```python
from build123d import *

# Parameters (mm, degrees)
FR4_DEPTH                     = 1.7526
SKETCH6_W                     = 5.5
SKETCH6_H                     = 5
SKETCH6_W_2                   = 13.6
SKETCH6_H_2                   = 5.5
FIBER_TRANSCEIVER_SLOTS_DEPTH = 143.1375095
SKETCH7_R                     = 1.905
CUT_EXTRUDE1_DEPTH            = 143.1375095
SKETCH8_R                     = 3.175
CUT_EXTRUDE2_DEPTH            = 143.1375095
CUT_EXTRUDE3_DEPTH            = 143.1375095


with BuildPart() as part:
    # Sketch1 → FR4 (new body)
    with BuildSketch(Plane(origin=(0, 0, 0), x_dir=(1, 0, 0), z_dir=(0, 1, 0))):
        with BuildLine():
            Line((0, 0), (5, 0))
            ThreePointArc((5, 0), (6.414213562, -0.585786438), (7, -2))
            Line((7, -2), (7, -13))
            ThreePointArc((7, -13), (7.585786438, -14.414213562), (9, -15))
            Line((9, -15), (22.5, -15))
            ThreePointArc((22.5, -15), (23.914213562, -14.414213562), (24.5, -13))
            Line((24.5, -13), (24.5, -2))
            ThreePointArc((24.5, -2), (25.085786438, -0.585786438), (26.5, 0))
            Line((26.5, 0), (83.5, 0))
            ThreePointArc((83.5, 0), (84.914213562, -0.585786438), (85.5, -2))
            Line((85.5, -2), (85.5, -13))
            ThreePointArc((85.5, -13), (86.085786438, -14.414213562), (87.5, -15))
            Line((87.5, -15), (101, -15))
            ThreePointArc((101, -15), (102.414213562, -14.414213562), (103, -13))
            Line((103, -13), (103, -2))
            ThreePointArc((103, -2), (103.585786438, -0.585786438), (105, 0))
            Line((105, 0), (110, 0))
            Line((110, 0), (110, 88))
            ThreePointArc((110, 88), (109.414213562, 89.414213562), (108, 90))
            Line((108, 90), (2, 90))
            ThreePointArc((2, 90), (0.585786438, 89.414213562), (0, 88))
            Line((0, 88), (0, 0))
        make_face()
    extrude(amount=FR4_DEPTH)

    # Sketch6 → fiber-transceiver-slots (cut, through all)
    with BuildSketch(Plane(origin=(0, 1.7526, 0), x_dir=(1, 0, 0), z_dir=(0, 1, 0))):
        with Locations((16.25, 32)):
            Rectangle(SKETCH6_W, SKETCH6_H)
        with Locations((94.25, 32)):
            Rectangle(SKETCH6_W, SKETCH6_H)
        with Locations((94.3, 45.45)):
            Rectangle(SKETCH6_W_2, SKETCH6_H_2)
        with Locations((16.3, 45.45)):
            Rectangle(SKETCH6_W_2, SKETCH6_H_2)
    extrude(amount=-FIBER_TRANSCEIVER_SLOTS_DEPTH, mode=Mode.SUBTRACT)

    # Sketch7 → Cut-Extrude1 (cut, through all)
    with BuildSketch(Plane(origin=(0, 1.7526, 0), x_dir=(1, 0, 0), z_dir=(0, 1, 0))):
        with Locations(Location((3.5, 15, 0), (0, 0, 270))):
            Circle(SKETCH7_R)
        with Locations(Location((106.5, 15, 0), (0, 0, 270))):
            Circle(SKETCH7_R)
        with Locations(Location((106.5, 30, 0), (0, 0, 270))):
            Circle(SKETCH7_R)
        with Locations(Location((106.5, 45, 0), (0, 0, 270))):
            Circle(SKETCH7_R)
        with Locations(Location((106.5, 60, 0), (0, 0, 270))):
            Circle(SKETCH7_R)
        with Locations(Location((106.5, 75, 0), (0, 0, 270))):
            Circle(SKETCH7_R)
        with Locations(Location((3.5, 30, 0), (0, 0, 270))):
            Circle(SKETCH7_R)
        with Locations(Location((3.5, 45, 0), (0, 0, 270))):
            Circle(SKETCH7_R)
        with Locations(Location((3.5, 60, 0), (0, 0, 270))):
            Circle(SKETCH7_R)
        with Locations(Location((3.5, 75, 0), (0, 0, 270))):
            Circle(SKETCH7_R)
    extrude(amount=-CUT_EXTRUDE1_DEPTH, mode=Mode.SUBTRACT)

    # Sketch8 → Cut-Extrude2 (cut, through all)
    with BuildSketch(Plane(origin=(0, 1.7526, 0), x_dir=(1, 0, 0), z_dir=(0, 1, 0))):
        with Locations(Location((3.5, 30, 0), (0, 0, 270))):
            Circle(SKETCH8_R)
        with Locations(Location((3.5, 60, 0), (0, 0, 270))):
            Circle(SKETCH8_R)
        with Locations(Location((106.5, 60, 0), (0, 0, 270))):
            Circle(SKETCH8_R)
        with Locations(Location((106.5, 30, 0), (0, 0, 270))):
            Circle(SKETCH8_R)
    extrude(amount=-CUT_EXTRUDE2_DEPTH, mode=Mode.SUBTRACT)

    # Sketch9 → Cut-Extrude3 (cut, through all)
    with BuildSketch(Plane(origin=(0, 1.7526, 0), x_dir=(1, 0, 0), z_dir=(0, 1, 0))):
        with BuildLine():
            Line((0, 63.175), (3.5, 63.175))
            ThreePointArc((3.5, 63.175), (6.675, 60), (3.5, 56.825))
            Line((3.5, 56.825), (0, 56.825))
            Line((0, 56.825), (0, 63.175))
        make_face()
        with BuildLine():
            Line((0, 33.175), (3.5, 33.175))
            ThreePointArc((3.5, 33.175), (6.675, 30), (3.5, 26.825))
            Line((3.5, 26.825), (0, 26.825))
            Line((0, 26.825), (0, 33.175))
        make_face()
        with BuildLine():
            Line((110, 63.175), (106.5, 63.175))
            ThreePointArc((106.5, 63.175), (103.325, 60), (106.5, 56.825))
            Line((106.5, 56.825), (110, 56.825))
            Line((110, 56.825), (110, 63.175))
        make_face()
        with BuildLine():
            Line((110, 33.175), (106.5, 33.175))
            ThreePointArc((106.5, 33.175), (103.325, 30), (106.5, 26.825))
            Line((106.5, 26.825), (110, 26.825))
            Line((110, 26.825), (110, 33.175))
        make_face()
    extrude(amount=-CUT_EXTRUDE3_DEPTH, mode=Mode.SUBTRACT)


solid = part.part
```
Verification items for the finished model (mm, model axes). Give positions to 0.01 mm unless a question says otherwise; leave off trailing zeros. Loops run counter-clockwise (first coordinate to the right, second up) from the corner with the lowest first, then second, coordinate; pieces in that order, holes last.
1. Go/stop test with flat-tipped pins: pin 1 Ø0.9 at (x, y) = (2.5, 1) entering from +Z; pin 2 Ø0.5 at (y, z) = (1, 8) entering from +X. Record where each tip stops, or that it passes through.
2. Thickness scan on line 1 (X direction, y = 0.75, z = -75) (3 decimals); line 2 (X direction, y = 0.5, z = -45) (3 decimals); line 3 (Z direction, x = 15.5, y = 1.4). Record the ranges inside material, lowest first.
3. Section check B-B, the plane x = 90. Enter the section's corners in (y, z), then the cut area to 3 significant figures.
4. Section check C-C, the plane z = -45. Enter the section's corners in (x, y) (3 decimals).
5. Mould release check, pull along Z, two halves, no side actions. Record for faces 1 (the flat face through (54, 0, -38)), 2 (the cylindrical face through (103.326, 0.889, -60.07)): released by +Z, released by -Z, zero draft, split by the parting line, or undercut.
6. Section check D-D, the plane y = 1. Count the separate pieces of the cut face and the enclosed holes in it, then the cut area to 4 significant figures.
7. Section check A-A, the plane z = -15. Enter the section's corners in (x, y) (3 decimals), then the cut area to 3 significant figures.
Geometry says:
1. pin 1: stops at z = 0
1. pin 2: stops at x = 103
2. line 1: x = 0 to 1.595, 5.405 to 104.595, 108.405 to 110
2. line 2: x = 0 to 1.595, 5.405 to 9.5, 23.1 to 87.5, 101.1 to 104.595, 108.405 to 110
2. line 3: z = -90 to -48.2, -42.7 to -34.5, -29.5 to 15
3. outline: (0, -90) - (1.75, -90) - (1.75, -48.2) - (0, -48.2) - close; (0, -42.7) - (1.75, -42.7) - (1.75, 15) - (0, 15) - close
3. area: 174 mm2
4. outline: (0, 0) - (1.595, 0) - (1.595, 1.753) - (0, 1.753) - close; (5.405, 0) - (9.5, 0) - (9.5, 1.753) - (5.405, 1.753) - close; (23.1, 0) - (87.5, 0) - (87.5, 1.753) - (23.1, 1.753) - close; (101.1, 0) - (104.595, 0) - (104.595, 1.753) - (101.1, 1.753) - close; (108.405, 0) - (110, 0) - (110, 1.753) - (108.405, 1.753) - close
5. face 1: zero draft
5. face 2: undercut
6. separate pieces: 1
6. enclosed holes: 10
6. area: 10,000 mm2
7. outline: (0, 0) - (1.595, 0) - (1.595, 1.753) - (0, 1.753) - close; (5.405, 0) - (104.595, 0) - (104.595, 1.753) - (5.405, 1.753) - close; (108.405, 0) - (110, 0) - (110, 1.753) - (108.405, 1.753) - close
7. area: 179 mm2
